Part model, mm, in its own coordinate system. A direction names the side the tool comes from. Coordinates: 2 decimals unless noted, no trailing zeros. Write each loop counter-clockwise with the first axis right and the second up, starting at its lowest first coordinate (ties: lowest second). Pieces come first, ordered by that corner, then holes. Notation, with made-up numbers: (27.25, -15.5) - (75.25, -15.5) arc R20 ccw to (75.25, -11.5) - close; hole circle Ø1 at (-10, -31.75). An arc over 180 degrees is marked (long way). Write each question's results on one line, items separated by ' | '.
from build123d import *

# Parameters (mm, degrees)
SKETCH3_R           = 59.15
SKETCH3_R_2         = 38.25
BOSS_EXTRUDE1_DEPTH = 40
SKETCH4_R           = 41.021
CUT_EXTRUDE1_DEPTH  = 3.556
SKETCH5_R           = 50.8
BOSS_EXTRUDE2_DEPTH = 2
SKETCH7_R           = 44.45
BOSS_EXTRUDE3_DEPTH = 7.366
CUT_EXTRUDE2_DEPTH  = 2.794
BOSS_EXTRUDE5_DEPTH = 13.91
SKETCH11_R          = 41.021
BOSS_EXTRUDE6_DEPTH = 4.318
SKETCH12_R          = 8
BOSS_EXTRUDE7_DEPTH = 50


with BuildPart() as part:
    # Sketch3 → Boss-Extrude1 (new body)
    with BuildSketch(Plane(origin=(0, 0, 0), x_dir=(1, 0, 0), z_dir=(0, 1, 0))):
        with Locations(Location((0, 0, 0), (0, 0, 270))):
            Circle(SKETCH3_R)
        with Locations(Location((0, 0, 0), (0, 0, 270))):
            Circle(SKETCH3_R_2, mode=Mode.SUBTRACT)
    extrude(amount=BOSS_EXTRUDE1_DEPTH)

    # Sketch4 → Cut-Extrude1 (cut)
    with BuildSketch(Plane(origin=(0, 40, 0), x_dir=(1, 0, 0), z_dir=(0, 1, 0))):
        with Locations(Location((0, 0, 0), (0, 0, 270))):
            Circle(SKETCH4_R)
    cut_extrude1 = extrude(amount=-CUT_EXTRUDE1_DEPTH, mode=Mode.SUBTRACT)

    # Mirror1: Cut-Extrude1 across plane
    add(cut_extrude1.mirror(Plane.ZX.offset(20)), mode=Mode.SUBTRACT)



with BuildPart() as body_2:
    # Sketch5 → Boss-Extrude2 (new body)
    with BuildSketch(Plane(origin=(0, 40, 0), x_dir=(1, 0, 0), z_dir=(0, 1, 0))):
        with Locations(Location((0, 0, 0), (0, 0, 270))):
            Circle(SKETCH5_R)
    extrude(amount=BOSS_EXTRUDE2_DEPTH)

    # Sketch7 → Boss-Extrude3 (add)
    with BuildSketch(Plane(origin=(0, 42, 0), x_dir=(1, 0, 0), z_dir=(0, 1, 0))):
        with Locations(Location((0, 0, 0), (0, 0, 270))):
            Circle(SKETCH7_R)
    extrude(amount=-BOSS_EXTRUDE3_DEPTH)

    # Sketch8 → Cut-Extrude2 (cut)
    with BuildSketch(Plane(origin=(0, 42, 0), x_dir=(1, 0, 0), z_dir=(0, 1, 0))):
        with BuildLine():
            Line((-3.717986915, 11.786271444), (-12.545239758, 39.769263451))
            ThreePointArc((-12.545239758, 39.769263451), (-12.171377231, 42.035175802), (-10.12290422, 43.073390757))
            Line((-10.12290422, 43.073390757), (10.12290422, 43.073390757))
            ThreePointArc((10.12290422, 43.073390757), (12.171377231, 42.035175802), (12.545239758, 39.769263451))
            Line((12.545239758, 39.769263451), (3.832946747, 12.150701932))
            ThreePointArc((3.832946747, 12.150701932), (5.461454635, 9.696711292), (8.348217029, 9.113006841))
            Line((8.348217029, 9.113006841), (28.16857256, 30.749128053))
            ThreePointArc((28.16857256, 30.749128053), (30.317841482, 31.558309782), (32.241198512, 30.303387593))
            Line((32.241198512, 30.303387593), (42.364102732, 12.770003164))
            ThreePointArc((42.364102732, 12.770003164), (42.489218712, 10.47686602), (40.713812318, 9.020135398))
            Line((40.713812318, 9.020135398), (12.43928992, 2.755921712))
            ThreePointArc((12.43928992, 2.755921712), (11.12832563, 0.11859719), (12.066203944, -2.673264603))
            Line((12.066203944, -2.673264603), (40.713812318, -9.020135398))
            ThreePointArc((40.713812318, -9.020135398), (42.489218712, -10.47686602), (42.364102732, -12.770003164))
            Line((42.364102732, -12.770003164), (32.241198512, -30.303387593))
            ThreePointArc((32.241198512, -30.303387593), (30.317841482, -31.558309782), (28.16857256, -30.749128053))
            Line((28.16857256, -30.749128053), (8.606343173, -9.39478022))
            ThreePointArc((8.606343173, -9.39478022), (5.666870994, -9.578114102), (3.717986915, -11.786271444))
            Line((3.717986915, -11.786271444), (12.545239758, -39.769263451))
            ThreePointArc((12.545239758, -39.769263451), (12.171377231, -42.035175802), (10.12290422, -43.073390757))
            Line((10.12290422, -43.073390757), (-10.12290422, -43.073390757))
            ThreePointArc((-10.12290422, -43.073390757), (-12.171377231, -42.035175802), (-12.545239758, -39.769263451))
            Line((-12.545239758, -39.769263451), (-3.832946747, -12.150701932))
            ThreePointArc((-3.832946747, -12.150701932), (-5.461454635, -9.696711292), (-8.348217029, -9.113006841))
            Line((-8.348217029, -9.113006841), (-28.16857256, -30.749128053))
            ThreePointArc((-28.16857256, -30.749128053), (-30.317841482, -31.558309782), (-32.241198512, -30.303387593))
            Line((-32.241198512, -30.303387593), (-42.364102732, -12.770003164))
            ThreePointArc((-42.364102732, -12.770003164), (-42.489218712, -10.47686602), (-40.713812318, -9.020135398))
            Line((-40.713812318, -9.020135398), (-12.43928992, -2.755921712))
            ThreePointArc((-12.43928992, -2.755921712), (-11.12832563, -0.11859719), (-12.066203944, 2.673264603))
            Line((-12.066203944, 2.673264603), (-40.713812318, 9.020135398))
            ThreePointArc((-40.713812318, 9.020135398), (-42.489218712, 10.47686602), (-42.364102732, 12.770003164))
            Line((-42.364102732, 12.770003164), (-32.241198512, 30.303387593))
            ThreePointArc((-32.241198512, 30.303387593), (-30.317841482, 31.558309782), (-28.16857256, 30.749128053))
            Line((-28.16857256, 30.749128053), (-8.606343173, 9.39478022))
            ThreePointArc((-8.606343173, 9.39478022), (-5.666870994, 9.578114102), (-3.717986915, 11.786271444))
        make_face()
    extrude(amount=-CUT_EXTRUDE2_DEPTH, mode=Mode.SUBTRACT)


with BuildPart() as part_1:
    add(part.part)

    add(body_2.part)  # Boss-Extrude5 merges body 2
    # Sketch10 → Boss-Extrude5 (add)
    with BuildSketch(Plane(origin=(0, 39.206, 0), x_dir=(1, 0, 0), z_dir=(0, 1, 0))):
        with BuildLine():
            Line((10.12290422, 45.613390757), (-10.12290422, 45.613390757))
            ThreePointArc((-10.12290422, 45.613390757), (-14.219850242, 43.536960847), (-14.967575297, 39.005136146))
            Line((-14.967575297, 39.005136146), (-6.471688132, 12.072595881))
            ThreePointArc((-6.471688132, 12.072595881), (-6.854928199, 11.827206148), (-7.29904471, 11.727961017))
            Line((-7.29904471, 11.727961017), (-26.295651132, 32.464868513))
            ThreePointArc((-26.295651132, 32.464868513), (-30.594188976, 34.083231971), (-34.440903038, 31.573387593))
            Line((-34.440903038, 31.573387593), (-44.563807258, 14.040003164))
            ThreePointArc((-44.563807258, 14.040003164), (-44.814039218, 9.453728876), (-41.263226429, 6.540267633))
            Line((-41.263226429, 6.540267633), (-13.691018788, 0.431651613))
            ThreePointArc((-13.691018788, 0.431651613), (-13.67012508, -0.022938888), (-13.80623453, -0.457177633))
            Line((-13.80623453, -0.457177633), (-41.263226429, -6.540267633))
            ThreePointArc((-41.263226429, -6.540267633), (-44.814039218, -9.453728876), (-44.563807258, -14.040003164))
            Line((-44.563807258, -14.040003164), (-34.440903038, -31.573387593))
            ThreePointArc((-34.440903038, -31.573387593), (-30.594188976, -34.083231971), (-26.295651132, -32.464868513))
            Line((-26.295651132, -32.464868513), (-7.219330657, -11.640944268))
            ThreePointArc((-7.219330657, -11.640944268), (-6.81519688, -11.850145036), (-6.507189821, -12.185138651))
            Line((-6.507189821, -12.185138651), (-14.967575297, -39.005136146))
            ThreePointArc((-14.967575297, -39.005136146), (-14.219850242, -43.536960847), (-10.12290422, -45.613390757))
            Line((-10.12290422, -45.613390757), (10.12290422, -45.613390757))
            ThreePointArc((10.12290422, -45.613390757), (14.219850242, -43.536960847), (14.967575297, -39.005136146))
            Line((14.967575297, -39.005136146), (6.471688132, -12.072595881))
            ThreePointArc((6.471688132, -12.072595881), (6.854928199, -11.827206148), (7.29904471, -11.727961017))
            Line((7.29904471, -11.727961017), (26.295651132, -32.464868513))
            ThreePointArc((26.295651132, -32.464868513), (30.594188976, -34.083231971), (34.440903038, -31.573387593))
            Line((34.440903038, -31.573387593), (44.563807258, -14.040003164))
            ThreePointArc((44.563807258, -14.040003164), (44.814039218, -9.453728876), (41.263226429, -6.540267633))
            Line((41.263226429, -6.540267633), (13.691018788, -0.431651613))
            ThreePointArc((13.691018788, -0.431651613), (13.67012508, 0.022938888), (13.80623453, 0.457177633))
            Line((13.80623453, 0.457177633), (41.263226429, 6.540267633))
            ThreePointArc((41.263226429, 6.540267633), (44.814039218, 9.453728876), (44.563807258, 14.040003164))
            Line((44.563807258, 14.040003164), (34.440903038, 31.573387593))
            ThreePointArc((34.440903038, 31.573387593), (30.594188976, 34.083231971), (26.295651132, 32.464868513))
            Line((26.295651132, 32.464868513), (7.219330657, 11.640944268))
            ThreePointArc((7.219330657, 11.640944268), (6.81519688, 11.850145036), (6.507189821, 12.185138651))
            Line((6.507189821, 12.185138651), (14.967575297, 39.005136146))
            ThreePointArc((14.967575297, 39.005136146), (14.219850242, 43.536960847), (10.12290422, 45.613390757))
        make_face()
    extrude(amount=-BOSS_EXTRUDE5_DEPTH)

    # Sketch11 → Boss-Extrude6 (add)
    with BuildSketch(Plane.XZ.offset(-3.556)):
        with Locations(Location((0, 0, 0), (0, 0, 90))):
            Circle(SKETCH11_R)
    extrude(amount=BOSS_EXTRUDE6_DEPTH)

    # Sketch12 → Boss-Extrude7 (add)
    with BuildSketch(Plane.XZ.offset(0.762)):
        with Locations(Location((0, 0, 0), (0, 0, 270))):
            Circle(SKETCH12_R)
    extrude(amount=BOSS_EXTRUDE7_DEPTH)


solid = part_1.part
(1) Saw through at C-C on y = 11.5. Write the cut outline in (x, z), then the cut area to 3 significant figures.
Return value:
outline: circle Ø118.3 at (0, 0); hole circle Ø76.5 at (0, 0) | area: 6,400 mm^2
(2) Two-plate mould, pull along Y, no slides. Class faces 1 (the flat face through (15.7, 30, -20.9)), 2 (the flat face through (44, 40, 26)), 3 (the flat face through (8.07, 40.62, 25.58)): released by +Y, released by -Y, zero draft, split by the parting line, or undercut.
Return value:
face 1: undercut | face 2: released by +Y | face 3: zero draft
(3) Saw through at B-B on y = 29.5. Write the cut outline in (x, z).
Return value:
outline: circle Ø118.3 at (0, 0); hole (-37.81, -5.78) - (-13.69, -0.43) arc R1.31 ccw to (-13.81, 0.46) - (-37.81, 5.78) arc R38.25 ccw to start; hole (-23.91, -29.86) arc R38.25 ccw to (-13.9, -35.63) - (-6.47, -12.07) arc R1.31 ccw to (-7.3, -11.73) - close; hole (-23.91, 29.86) - (-7.22, 11.64) arc R1.31 ccw to (-6.51, 12.19) - (-13.9, 35.63) arc R38.25 ccw to start; hole (6.47, 12.07) arc R1.31 ccw to (7.3, 11.73) - (23.91, 29.86) arc R38.25 ccw to (13.9, 35.63) - close; hole (6.51, -12.19) - (13.9, -35.63) arc R38.25 ccw to (23.91, -29.86) - (7.22, -11.64) arc R1.31 ccw to start; hole (13.69, 0.43) arc R1.31 ccw to (13.81, -0.46) - (37.81, -5.78) arc R38.25 ccw to (37.81, 5.78) - close
(4) Saw through at A-A on x = 0. Write the cut outline in (y, z), then the cut area to 3 significant figures.
Return value:
outline: (-50.76, -8) - (-0.76, -8) - (-0.76, -41.02) - (0, -41.02) - (0, -59.15) - (40, -59.15) - (40, -50.8) - (42, -50.8) - (42, -43.07) - (40, -43.07) - (40, -41.02) - (39.21, -41.02) - (39.21, 41.02) - (40, 41.02) - (40, 43.07) - (42, 43.07) - (42, 50.8) - (40, 50.8) - (40, 59.15) - (0, 59.15) - (0, 41.02) - (-0.76, 41.02) - (-0.76, 8) - (-50.76, 8) - close; hole (3.56, -38.25) - (25.3, -38.25) - (25.3, 38.25) - (3.56, 38.25) - close | area: 3,900 mm^2
(5) Wall check: line 1 (X direction, y = 28.5, z = 0); line 2 (X direction, y = 19.5, z = 0); line 3 (Y direction, x = -17.5, z = -29). Give the ranges that are in metal, low to high. Write a range as from..to.
Return value:
line 1: x = -59.15..-38.25, -13.67..13.67, 38.25..59.15 | line 2: x = -59.15..-38.25, 38.25..59.15 | line 3: y = -0.76..3.56, 34.63..42
(6) Saw through at D-D on y = -31.5. Write the cut outline in (x, z), then the cut area to 3 significant figures.
Return value:
outline: circle Ø16 at (0, 0) | area: 201 mm^2
(7) 3-axis set-ups, long thin cutter, end or side, ignore diameter. For faces 4 (the flat face through (36, 40, 21)), 5 (the flat face through (-1, 3.556, -1)), 6 (the cylindrical face through (24.961, -0.376, -32.553)): which of +Z, -Z, +X, -X, +Y, -Y reach the whole face in a straight line?
Return value:
face 4: +Y | face 5: none | face 6: -Y
(8) Flat gauge pins, fed straight in: P1, Ø8.5, axis at x = -14, z = -27.5, coming from the -Y side; P2, Ø2, axis at x = -5, z = -41, coming from the +Y side; P3, Ø1, axis at y = 19, z = -29.5, coming from the +X side. Where does each tip first touch, or does it go through?
Return value:
P1: stops at y = -0.76 | P2: stops at y = 40 | P3: stops at x = 51.55
